from build123d import *

# Parameters (mm, degrees)
BOSS_EXTRUDE1_DEPTH = 50
VARFILLET1_R        = 10


with BuildPart() as part:
    # Sketch1 → Boss-Extrude1 (new body)
    with BuildSketch(Plane(origin=(0, 0, 0), x_dir=(1, 0, 0), z_dir=(0, 1, 0))):
        Polygon((0, 0), (49.1370117, 0), (49.1370117, 35.13023464), (35, 35.13023464), (35, 10.869893229), (0, 10.869893229), align=None)
    extrude(amount=BOSS_EXTRUDE1_DEPTH)

    # VarFillet1
    varfillet1_edges = [part.edges().sort_by_distance(p)[0] for p in [
        (35, 25, -10.869893229),
    ]]
    fillet(varfillet1_edges, radius=VARFILLET1_R)


solid = part.part
Verification items for the finished model (mm, model axes). A direction names the side the tool comes from. Give positions to 0.01 mm unless a question says otherwise; leave off trailing zeros. Loops run counter-clockwise (first coordinate to the right, second up) from the corner with the lowest first, then second, coordinate; pieces in that order, holes last.
1) Sectioned sample at A-A, the plane y = 4.5. Enter the section's corners in (x, z).
2) Sectioned sample at C-C, the plane z = -29. Enter the section's corners in (x, y).
3) Thickness scan on line 1 along Z through (x, y) = (12, 15); line 2 along X through (y, z) = (6, -21); line 3 along X through (y, z) = (28, -19). Record the ranges inside material, lowest first.
4) Sectioned sample at B-B, the plane x = 4.5. Enter the section's corners in (y, z).
5) Set-up check for faces 1 (the flat face through (30, 50, -10)), 2 (the flat face through (13, 25, -10.87)): record each of +Z, -Z, +X, -X, +Y, -Y from which the full face is reachable in a straight line by a thin tool's end or side.
6) Depth check by flat-ended pin: pin 1 Ø8 at (x, y) = (19, 39.5) entering from -Z; pin 2 Ø4.5 at (y, z) = (34, -28) entering from -X. Enter the tip coordinate at first touch or a pass-through.
Answers:
1. outline: (0, -10.87) - (25, -10.87) arc R10 cw to (35, -20.87) - (35, -35.13) - (49.14, -35.13) - (49.14, 0) - (0, 0) - close
2. outline: (35, 0) - (49.14, 0) - (49.14, 50) - (35, 50) - close
3. line 1: z = -10.87 to 0
3. line 2: x = 35 to 49.14
3. line 3: x = 34.82 to 49.14
4. outline: (0, -10.87) - (50, -10.87) - (50, 0) - (0, 0) - close
5. face 1: +Z, -Z, +X, -X, +Y
5. face 2: -Z, -X, +Y, -Y
6. pin 1: stops at z = -10.87
6. pin 2: stops at x = 35
